Source: three-view drawing plus pictorial views. Frame: mm from the lowest corner of the part. Coordinates: 2 decimals unless noted, no trailing zeros. Write each loop counter-clockwise with the first axis right and the second up, starting at its lowest first coordinate (ties: lowest second). Pieces come first, ordered by that corner, then holes. Notation, with made-up numbers: (-11.75, 60.5) - (6.25, 60.5) arc R19 cw to (6.25, 86.5) - close; hole circle Ø3 at (41.25, 30.5). An arc over 180 degrees is marked (long way). Put each result on its own line as item: value. Start each with the question number.
1. Line query: line 1 (X direction, y = 1.1, z = 51.77); line 2 (X direction, y = 1.45, z = 28.2); line 3 (Z direction, x = 28.5, y = 2.9). Output: solid intervals per line, ascending.
2. Cut plane D-D, the plane z = 51.77. Return loops of the section in (x, y).
3. Pin query (flat end, axial travel): pin 1 (3 mm diameter, centred on x = 19, y = 3, fed in from -Z); pin 2 (3 mm diameter, centred on x = 2.5, z = 51.77, fed in from -Y). Return the tip coordinate at first contact, or that it passes through.
4. Cut plane A-A, the plane x = 33.2. Return loops of the section in (y, z), and give its area (3 significant figures).
5. Cut plane B-B, the plane x = 63.9. Return loops of the section in (y, z).
6. Cut plane C-C, the plane y = 4.3. Count the separate pieces of the cut face and the enclosed holes in it, and give its area (3 significant figures).
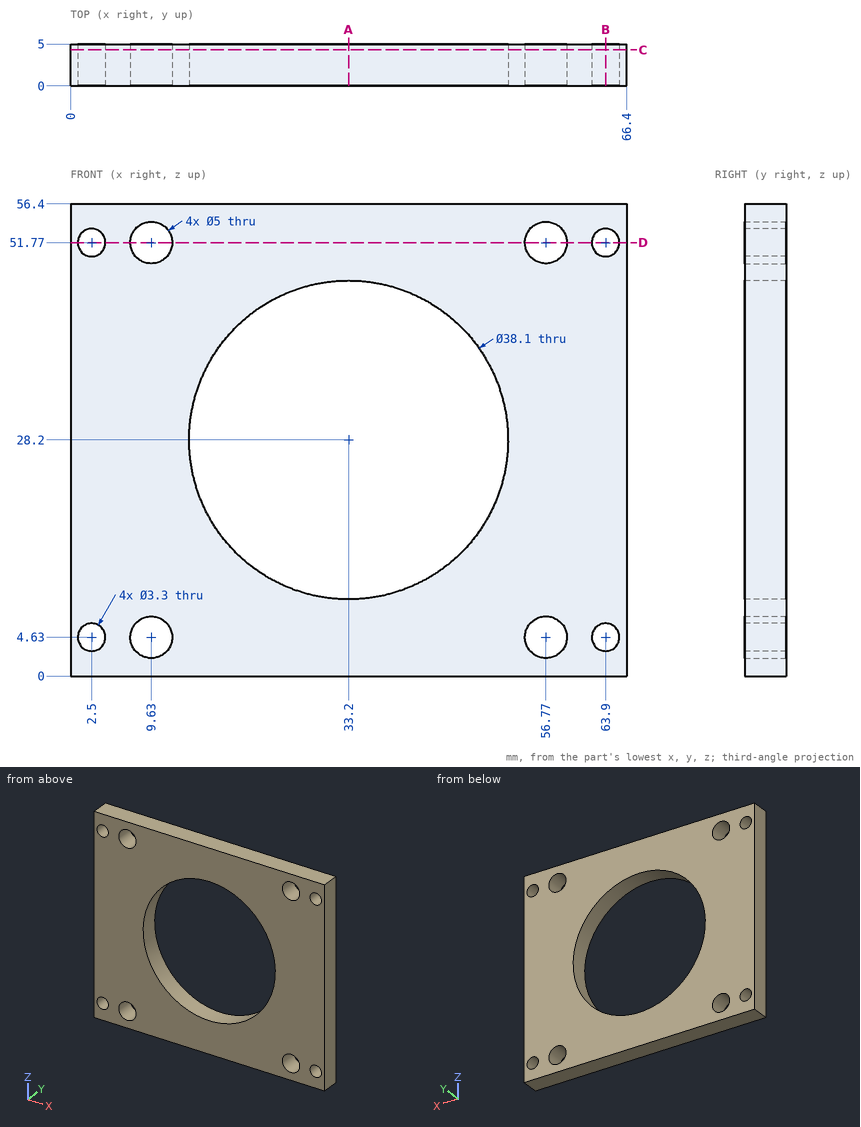
Report:
1. line 1: x = 0 to 0.85, 4.15 to 7.13, 12.13 to 54.27, 59.27 to 62.25, 65.55 to 66.4
1. line 2: x = 0 to 14.15, 52.25 to 66.4
1. line 3: z = 0 to 9.74, 46.66 to 56.4
2. outline: (0, 0) - (0.85, 0) - (0.85, 5) - (0, 5) - close; (4.15, 0) - (7.13, 0) - (7.13, 5) - (4.15, 5) - close; (12.13, 0) - (54.27, 0) - (54.27, 5) - (12.13, 5) - close; (59.27, 0) - (62.25, 0) - (62.25, 5) - (59.27, 5) - close; (65.55, 0) - (66.4, 0) - (66.4, 5) - (65.55, 5) - close
3. pin 1: stops at z = 0
3. pin 2: passes through
4. outline: (0, 0) - (5, 0) - (5, 9.15) - (0, 9.15) - close; (0, 47.25) - (5, 47.25) - (5, 56.4) - (0, 56.4) - close
4. area: 91.5 mm^2
5. outline: (0, 0) - (5, 0) - (5, 2.98) - (0, 2.98) - close; (0, 6.28) - (5, 6.28) - (5, 50.12) - (0, 50.12) - close; (0, 53.42) - (5, 53.42) - (5, 56.4) - (0, 56.4) - close
6. separate pieces: 1
6. enclosed holes: 9
6. area: 2,490 mm^2
